Here's how the part is built. I have some questions about the finished solid (model axes, mm). A direction names the side the tool comes from. Give positions to 0.01 mm unless a question says otherwise; leave off trailing zeros. Order: outer loops, then holes, each group sorted by start corner. A loop starts at its lowest first (then second) coordinate and runs counter-clockwise, first axis right, second up. Notation, with made-up numbers: M -18.5,-31.75 L 27.5,-31.75 A8 ccw 27.5,-19.75 Z; hole C 66.25,-26.5 d2. An arc over 180 degrees is marked long. Use one line per item in the form item = value.
from build123d import *

# Parameters (mm, degrees)
ESQUISSE1_R        = 26.257549031
ESQUISSE1_R_2      = 1.55
BOSS_EXTRU_1_DEPTH = 6


with BuildPart() as part:
    # Esquisse1 → Boss.-Extru.1 (new body)
    with BuildSketch(Plane.ZY):
        with Locations((16.097760006, -58.545962001)):
            Circle(ESQUISSE1_R)
        with Locations((29.226534372, -58.545962001)):
            Circle(ESQUISSE1_R_2, mode=Mode.SUBTRACT)
        with Locations((16.097760006, -45.417187634)):
            Circle(ESQUISSE1_R_2, mode=Mode.SUBTRACT)
        with Locations((2.968985639, -58.545962001)):
            Circle(ESQUISSE1_R_2, mode=Mode.SUBTRACT)
        with Locations((16.097760006, -71.674736367)):
            Circle(ESQUISSE1_R_2, mode=Mode.SUBTRACT)
        Polygon((16.097760006, -51.040408501), (9.597760006, -54.793185251), (9.597760006, -62.29873875), (16.097760006, -66.0515155), (22.597760006, -62.29873875), (22.597760006, -54.793185251), align=None, mode=Mode.SUBTRACT)
    extrude(amount=BOSS_EXTRU_1_DEPTH)


solid = part.part
Q1. Thinking about a two-plate mould opening in Z: for faces 3 (the face through (-2.96, -84.18, 10.41)), 4 (the face through (0, -64, 22)), 5 (the face through (-2.96, -52.94, 19.39)), which applies, +Z half, -Z half, draft (parallel to the pull), parting line (faces both ways), or undercut?
Found:
face_3 = parting line
face_4 = draft
face_5 = undercut
Q2. I want a section at A-A on x = -4.5. Write out the boundary of the cut face in (y, z), then the cut area to 3 significant figures.
Found:
outline = C -58.55,16.1 d52.52; hole C -71.67,16.1 d3.1; hole M -66.05,16.1 L -62.3,9.6 L -54.79,9.6 L -51.04,16.1 L -54.79,22.6 L -62.3,22.6 Z; hole C -58.55,2.97 d3.1; hole C -58.55,29.23 d3.1; hole C -45.42,16.1 d3.1
area = 1,990 mm²
Q3. On a 3-axis mill with a long thin cutter (end or side, diameter ignored), from which of +Z, -Z, +X, -X, +Y, -Y can I reach the whole of each face in a straight line? I mean faces 1 (the face through (-6, -64, 22)), 2 (the face through (-3, -58, 9.598)). Say none if no direction works.
Found:
face_1 = +Z, -Z, -X, +Y, -Y
face_2 = +X, -X
Q4. I want a section at B-B on z = 38.5. Write out the boundary of the cut face in (x, y).
Found:
outline = M -6,-72.24 L 0,-72.24 L 0,-44.85 L -6,-44.85 Z
Q5. I'm going to push flat-ended pins straight in: pin 1 Ø1 at (x, y) = (-2, -47.5) entering from +Z; pin 2 Ø2 at (x, y) = (-1.5, -45.5) entering from +Z; pin 3 Ø3 at (x, y) = (-2.5, -40.5) entering from -Z. Where does each tip first touch, or does it pass through?
Found:
pin_1 = 40.14
pin_2 = 39.43
pin_3 = -4.29
Q6. I want a section at C-C on y = -50. Write out the boundary of the cut face in (x, z), then the cut area to 3 significant figures.
Found:
outline = M -6,-8.73 L 0,-8.73 L 0,40.93 L -6,40.93 Z
area = 298 mm²
Q7. I need wall thicknesses on L1, parallel to Y at x = -2.5, z = 16; L2, parallel to Z at x = -3.95, y = -61; L3, parallel to Z at x = -3.5, y = -66. Which ranges of each line are inside material? Lowest first, please.
Found:
L1 = -84.8 to -73.22, -70.13 to -66, -51.1 to -46.96, -43.87 to -32.29
L2 = -10.04 to 9.6, 22.6 to 42.24
L3 = -9.08 to 16.01, 16.19 to 41.28
